Read the model definition and answer for the solid it produces. Units are mm, in the model's axes. A direction names the side the tool comes from. Coordinates: 2 decimals unless noted, no trailing zeros. Order: outer loops, then holes, each group sorted by start corner. A loop starts at its lowest first (then second) coordinate and runs counter-clockwise, first axis right, second up.
```python
from build123d import *

# Parameters (mm, degrees)
SKETCH1_R           = 17.5
SKETCH2_R           = 25
SHELL1_T            = -2
SKETCH3_R           = 7.25
SKETCH3_R_2         = 3
BOSS_EXTRUDE1_DEPTH = 5
CUT_EXTRUDE1_START  = -5
SKETCH4_R           = 3
CUT_EXTRUDE1_DEPTH  = 5
SKETCH5_R           = 1.5
CUT_EXTRUDE2_DEPTH  = 37.249138081
CUT_EXTRUDE3_DEPTH  = 15


with BuildPart() as part:
    # Sketch1 → Loft1 section 0
    with BuildSketch(Plane(origin=(0, 0, 0), x_dir=(1, 0, 0), z_dir=(0, 1, 0))):
        Circle(SKETCH1_R)
    # Sketch2 → Loft1 section 1
    with BuildSketch(Plane(origin=(0, 8, 0), x_dir=(1, 0, 0), z_dir=(0, 1, 0))):
        Circle(SKETCH2_R)
    loft()

    # Shell1
    shell1_openings = [part.faces().sort_by_distance(p)[0] for p in [
        (0, 8, 0),
    ]]
    offset(amount=SHELL1_T, openings=shell1_openings, kind=Kind.INTERSECTION)

    # Sketch3 → Boss-Extrude1 (add)
    with BuildSketch(Plane.XZ):
        with Locations(Location((0, 0, 0), (0, 0, 90))):
            Circle(SKETCH3_R)
        with Locations(Location((0, 0, 0), (0, 0, 270))):
            Circle(SKETCH3_R_2, mode=Mode.SUBTRACT)
    extrude(amount=BOSS_EXTRUDE1_DEPTH)

    # Sketch4 → Cut-Extrude1 (cut)
    with BuildSketch(Plane.XZ.offset(CUT_EXTRUDE1_START)):
        with Locations(Location((0, 0, 0), (0, 0, 90))):
            Circle(SKETCH4_R)
    extrude(amount=CUT_EXTRUDE1_DEPTH, mode=Mode.SUBTRACT)

    # Sketch5 → Cut-Extrude2 (cut, through all)
    with BuildSketch(Plane.XZ):
        with Locations(Location((0, 10, 0), (0, 0, 270))):
            Circle(SKETCH5_R)
        with Locations(Location((8.660254038, -5, 0), (0, 0, 270))):
            Circle(SKETCH5_R)
        with Locations(Location((-8.660254038, -5, 0), (0, 0, 270))):
            Circle(SKETCH5_R)
    extrude(amount=-CUT_EXTRUDE2_DEPTH, mode=Mode.SUBTRACT)

    # Sketch6 → Cut-Extrude3 (cut)
    with BuildSketch(Plane.XZ.offset(5)):
        with BuildLine():
            Line((-5.012820513, 16.230769231), (-5.846153846, 18.230769231))
            ThreePointArc((-5.846153846, 18.230769231), (-5.664100589, 20.109400392), (-4, 21))
            Line((-4, 21), (4, 21))
            ThreePointArc((4, 21), (5.664100589, 20.109400392), (5.846153846, 18.230769231))
            Line((5.846153846, 18.230769231), (5.012820513, 16.230769231))
            ThreePointArc((5.012820513, 16.230769231), (4.276067059, 15.335899411), (3.166666667, 15))
            Line((3.166666667, 15), (-3.166666667, 15))
            ThreePointArc((-3.166666667, 15), (-4.276067059, 15.335899411), (-5.012820513, 16.230769231))
        make_face()
        with BuildLine():
            Line((15, -3.166666667), (15, 3.166666667))
            ThreePointArc((15, 3.166666667), (15.335899411, 4.276067059), (16.230769231, 5.012820513))
            Line((16.230769231, 5.012820513), (18.230769231, 5.846153846))
            ThreePointArc((18.230769231, 5.846153846), (20.109400392, 5.664100589), (21, 4))
            Line((21, 4), (21, -4))
            ThreePointArc((21, -4), (20.109400392, -5.664100589), (18.230769231, -5.846153846))
            Line((18.230769231, -5.846153846), (16.230769231, -5.012820513))
            ThreePointArc((16.230769231, -5.012820513), (15.335899411, -4.276067059), (15, -3.166666667))
        make_face()
        with BuildLine():
            Line((-3.166666667, -15), (3.166666667, -15))
            ThreePointArc((3.166666667, -15), (4.276067059, -15.335899411), (5.012820513, -16.230769231))
            Line((5.012820513, -16.230769231), (5.846153846, -18.230769231))
            ThreePointArc((5.846153846, -18.230769231), (5.664100589, -20.109400392), (4, -21))
            Line((4, -21), (-4, -21))
            ThreePointArc((-4, -21), (-5.664100589, -20.109400392), (-5.846153846, -18.230769231))
            Line((-5.846153846, -18.230769231), (-5.012820513, -16.230769231))
            ThreePointArc((-5.012820513, -16.230769231), (-4.276067059, -15.335899411), (-3.166666667, -15))
        make_face()
        with BuildLine():
            Line((-15, 3.166666667), (-15, -3.166666667))
            ThreePointArc((-15, -3.166666667), (-15.335899411, -4.276067059), (-16.230769231, -5.012820513))
            Line((-16.230769231, -5.012820513), (-18.230769231, -5.846153846))
            ThreePointArc((-18.230769231, -5.846153846), (-20.109400392, -5.664100589), (-21, -4))
            Line((-21, -4), (-21, 4))
            ThreePointArc((-21, 4), (-20.109400392, 5.664100589), (-18.230769231, 5.846153846))
            Line((-18.230769231, 5.846153846), (-16.230769231, 5.012820513))
            ThreePointArc((-16.230769231, 5.012820513), (-15.335899411, 4.276067059), (-15, 3.166666667))
        make_face()
    extrude(amount=-CUT_EXTRUDE3_DEPTH, mode=Mode.SUBTRACT)


solid = part.part
```
1) A cutting plane is placed at A-A, the plane y = -1.5. Determine the outline of the cut face in (x, z), and give its area (3 significant figures).
A:
outline: circle Ø14.5 at (0, 0); hole circle Ø6 at (0, 0)
area: 137 mm2
2) Straight lines are drawn through the part: line 1 (X direction, y = 0.8, z = -5); line 2 (X direction, y = -3, z = 0); line 3 (Y direction, x = -4, z = 7.5). For each, find the intervals that lie inside material, in ascending order.
A:
line 1: x = -16.2 to -10.16, -7.16 to 7.16, 10.16 to 16.2
line 2: x = -7.25 to -3, 3 to 7.25
line 3: y = 0 to 2
3) Flat-ended cylindrical pins translate along their axes: pin 1 Ø2.5 at (x, y) = (0, 5.5) entering from +Z; pin 2 Ø3.5 at (x, z) = (8.66, -5) entering from -Y; pin 3 Ø2 at (y, z) = (1.5, 0) entering from -X. Find the tip coordinate at first contact, or state that the pin passes through.
A:
pin 1: stops at z = 23.83
pin 2: stops at y = 0
pin 3: stops at x = -15
4) A cutting plane is placed at B-B, the plane x = 0. Determine the outline of the cut face in (y, z).
A:
outline: (-5, -7.25) - (0, -7.25) - (0, -15) - (2, -15) - (2, -3) - (-5, -3) - close; (-5, 3) - (2, 3) - (2, 8.5) - (0, 8.5) - (0, 7.25) - (-5, 7.25) - close; (0, 11.5) - (2, 11.5) - (2, 15) - (0, 15) - close; (3.73, -21) - (8, -25) - (8, -22.26) - (6.66, -21) - close; (3.73, 21) - (6.66, 21) - (8, 22.26) - (8, 25) - close
5) Determine the mould class of faces 1 (the cylindrical face through (-4.29, 1.172, -15.345)), 2 (the cylindrical face through (-4.262, 0.908, 15.327)), 3 (the cylindrical face through (0.07, 0.99, 11.5)) for opening direction Z: pulls with the +Z half, pulls with the -Z half, needs draft (parallel to the pull), parting line crosses it, or undercut.
A:
face 1: pulls with the -Z half
face 2: pulls with the +Z half
face 3: undercut
6) Which of the six approach directions +Z, -Z, +X, -X, +Y, -Y give full straight-line access (tool end or side, diameter ignored) to faces 4 (the flat face through (0, 2, -4)), 5 (the flat face through (0, 1, -15)), 6 (the cylindrical face through (-5.65, 4.99, -20.13)), 7 (the cylindrical face through (-15.345, 1.172, 4.29)), 8 (the cylindrical face through (15.345, 1.172, -4.29))?
A:
face 4: +Y
face 5: -Z, +Y, -Y
face 6: +Y, -Y
face 7: -X, +Y, -Y
face 8: +X, +Y, -Y
7) A cutting plane is placed at C-C, the plane z = 0. State how many separate pieces and enclosed holes the cut face has, and give its area (3 significant figures).
A:
separate pieces: 4
enclosed holes: 0
area: 106 mm2
